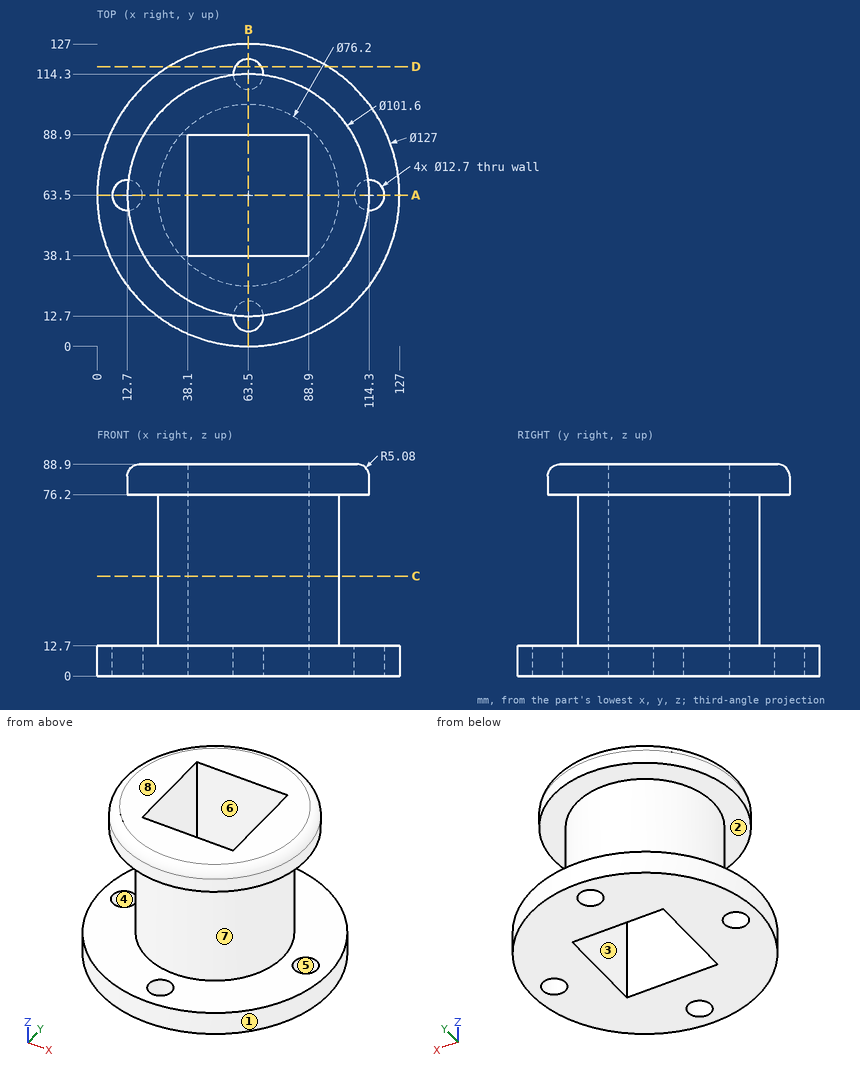
Design review of the part shown in the three views and the two pictorial views. Dimensions are in mm from the part's minimum x, y and z. A direction names the side the tool comes from. Round coordinates to 2 decimals unless told otherwise and drop trailing zeros. Write each loop counter-clockwise with the first axis right and the second up, starting at its lowest first coordinate (ties: lowest second). Pieces come first, ordered by that corner, then holes. Notation, with made-up numbers: M -23.5,72.25 L 23.5,72.25 A15 ccw 23.5,82.25 Z; hole C -18,42.5 d4. An arc over 180 degrees is marked long. One line per item, written item: value. Start each with the question number.
1. Take a section at C-C on z = 42. State the section outline as (x, y) points.
2. Clearance check with flat-ended pins moving along their axes: P1, Ø7.5, axis at x = 12.7, y = 63.5, coming from the -Z side; P2, Ø4, axis at y = 94, z = 19.5, coming from the +X side; P3, Ø1, axis at y = 98.5, z = 19, coming from the -X side. State where each tip first meets the part, or that it passes through.
3. To check wall thickness, follow probe 1 along X at (y, z) = (63, 6); probe 2 along Y at (x, z) = (63.5, 6.5); probe 3 along Z at (x, y) = (39, 96). State the ranges of each line that lie inside material, in increasing order. Write a range as from..to.
4. For the marked faces 5, 6, 7 and 8, list the 3-axis set-ups (+Z, -Z, +X, -X, +Y, -Y) from which the entire face can be reached by the end or side of a thin tool; tool diameter is ignored.
5. Take a section at A-A on y = 63.5. State the section outline as (x, z) points.
6. Take a section at D-D on y = 117.5. State the section outline as (x, z) points.
7. Draft analysis for pull direction Y (two halves, no side actions). For the marked faces 1, 2, 3 and 4, state which applies: pulls with the +Y half, pulls with the -Y half, needs draft (parallel to the pull), parting line crosses it, or undercut.
Computed:
1. outline: C 63.5,63.5 d76.2; hole M 38.1,38.1 L 88.9,38.1 L 88.9,88.9 L 38.1,88.9 Z
2. P1: stops at z = 76.2
2. P2: stops at x = 88.79
2. P3: stops at x = 47.33
3. probe 1: x = 0..6.37, 19.03..38.1, 88.9..107.97, 120.63..127
3. probe 2: y = 0..6.35, 19.05..38.1, 88.9..107.95, 120.65..127
3. probe 3: z = 0..12.7, 76.2..88.9
4. face 5: -Z
4. face 6: +Z, -Z
4. face 7: none
4. face 8: +Z, +X, -X, +Y, -Y
5. outline: M 0,0 L 6.35,0 L 6.35,12.7 L 0,12.7 Z; M 12.7,76.2 L 25.4,76.2 L 25.4,12.7 L 19.05,12.7 L 19.05,0 L 38.1,0 L 38.1,88.9 L 17.78,88.9 A5.08 ccw 12.7,83.82 Z; M 88.9,0 L 107.95,0 L 107.95,12.7 L 101.6,12.7 L 101.6,76.2 L 114.3,76.2 L 114.3,83.82 A5.08 ccw 109.22,88.9 L 88.9,88.9 Z; M 120.65,0 L 127,0 L 127,12.7 L 120.65,12.7 Z
6. outline: M 30.09,0 L 58.02,0 L 58.02,12.7 L 30.09,12.7 Z; M 68.98,0 L 96.91,0 L 96.91,12.7 L 68.98,12.7 Z
7. face 1: parting line crosses it
7. face 2: needs draft
7. face 3: undercut
7. face 4: undercut
